Here's how the part is built. I have some questions about the finished solid (model axes, mm). Face numbers are marked on the shaded views. A direction names the side the tool comes from. Round coordinates to 2 decimals unless told otherwise and drop trailing zeros. Order: outer loops, then holes, each group sorted by start corner. A loop starts at its lowest first (then second) coordinate and runs counter-clockwise, first axis right, second up.
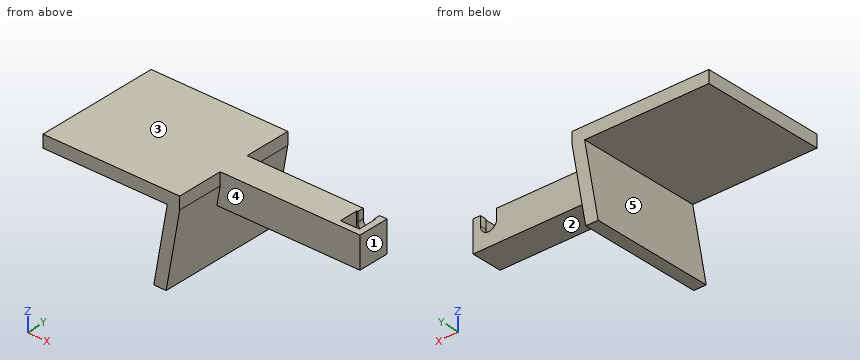
```python
from build123d import *

# Parameters (mm, degrees)
PAD001_DEPTH    = 20
SKETCH004_W     = 39
SKETCH004_H     = 10
PAD_DEPTH       = 10
SKETCH_W        = 10
SKETCH_H        = 10
PAD002_DEPTH    = 10
SKETCH001_W     = 6
SKETCH001_H     = 6
POCKET_DEPTH    = 6
POCKET001_DEPTH = 17.001


with BuildPart() as part:
    # Sketch003 → Pad001 (new body, symmetric)
    with BuildSketch(Plane(origin=(-40, 0, 0), x_dir=(1, 0, 0), z_dir=(0, -1, 0))):
        Polygon((0, 0), (-44, 0), (-44, -4), (-4, -4), (-8.341204, -28.620194), (-4.341204, -28.620194), (0, -4), align=None)
    extrude(amount=PAD001_DEPTH, both=True)

    # Sketch004 → Pad (join)
    with BuildSketch(Plane.XY):
        with Locations((-24.5, 0)):
            Rectangle(SKETCH004_W, SKETCH004_H)
    extrude(amount=-PAD_DEPTH)

    # Sketch → Pad002 (join)
    with BuildSketch(Plane.XY):
        Rectangle(SKETCH_W, SKETCH_H)
    extrude(amount=-PAD002_DEPTH)

    # Sketch001 → Pocket (cut)
    with BuildSketch(Plane.XY):
        Rectangle(SKETCH001_W, SKETCH001_H)
    extrude(amount=-POCKET_DEPTH, mode=Mode.SUBTRACT)

    # Sketch002 → Pocket001 (cut, through all)
    with BuildSketch(Plane.XZ.offset(-3)):
        with BuildLine():
            ThreePointArc((-2.625, -3), (0, -5.625), (2.625, -3))
            Line((2.625, -3), (2.625, 6))
            ThreePointArc((2.625, 6), (0, 8.625), (-2.625, 6))
            Line((-2.625, 6), (-2.625, -3))
        make_face()
    extrude(amount=-POCKET001_DEPTH, mode=Mode.SUBTRACT)


solid = part.part
```
1. On a 3-axis mill with a long thin cutter (end or side, diameter ignored), from which of +Z, -Z, +X, -X, +Y, -Y can I reach the whole of each face in a straight line? I mean the marked faces 1 and 2. Say none if no direction works.
Evaluation:
face 1: +Z, -Z, +X, +Y, -Y
face 2: -Z, +X, +Y, -Y
2. If we section it at D-D, the plane z = -26.5: Write out the boundary of the cut face in (x, y).
Evaluation:
outline: (-47.97, -20) - (-43.97, -20) - (-43.97, 20) - (-47.97, 20) - close
3. If we section it at C-C, the plane x = 0: Write out the boundary of the cut face in (y, z) (3 decimals).
Evaluation:
outline: (-5, -10) - (5, -10) - (5, -5.625) - (3, -5.625) - (3, -6) - (-3, -6) - (-3, 0) - (-5, 0) - close
4. If we section it at B-B, the plane y = -11: Write out the boundary of the cut face in (x, z).
Evaluation:
outline: (-84, -4) - (-44, -4) - (-48.34, -28.62) - (-44.34, -28.62) - (-40, -4) - (-40, 0) - (-84, 0) - close
5. I need wall thicknesses on probe 1 along Z at (x, y) = (-56.5, -10); probe 2 along Y at (x, z) = (-33, -4); probe 3 along Z at (x, y) = (-23, -2). Which ranges of each line are inside material? Lowest first, please.
Evaluation:
probe 1: z = -4 to 0
probe 2: y = -5 to 5
probe 3: z = -10 to 0
6. I'm going to push flat-ended pins straight in: P1, Ø8, axis at x = -25, z = -5, coming from the +Y side; P2, Ø4, axis at y = -15.5, z = -22.5, coming from the +X side; P3, Ø11, axis at x = -24, z = -4.5, coming from the -Y side. Where does each tip first touch, or does it pass through?
Evaluation:
P1: stops at y = 5
P2: stops at x = -42.91
P3: stops at y = -5
7. If we section it at A-A, the plane x = -46: Write out the boundary of the cut face in (y, z), and give its area (3 significant figures).
Evaluation:
outline: (-20, -28.62) - (20, -28.62) - (20, -15.34) - (-20, -15.34) - close; (-20, -4) - (20, -4) - (20, 0) - (-20, 0) - close
area: 691 mm2
8. If we mould it in two halves opening along Z, with no side actions, what happens to the marked faces 3, 4 and 5? For each: released by +Z, released by -Z, zero draft, split by the parting line, or undercut.
Evaluation:
face 3: released by +Z
face 4: zero draft
face 5: undercut
